Check sheet for the modelled part. Datum: model origin and axes. Units: mm. Round coordinates to 2 decimals unless told otherwise and drop trailing zeros. Write each loop counter-clockwise with the first axis right and the second up, starting at its lowest first coordinate (ties: lowest second). Pieces come first, ordered by that corner, then holes. Notation, with made-up numbers: (-21.5, 75.5) -> (7.5, 75.5) arc R18 ccw to (7.5, 81.5) -> close; hole circle Ø5 at (19, 6). An arc over 180 degrees is marked (long way). One line per item, written item: value.
from build123d import *

# Parameters (mm, degrees)
SALIENTE_EXTRUIR1_DEPTH = 10
SALIENTE_EXTRUIR2_DEPTH = 10
CROQUIS3_R              = 25
CORTAR_EXTRUIR1_DEPTH   = 10


with BuildPart() as part:
    # Croquis1 → Saliente-Extruir1 (new body)
    with BuildSketch(Plane(origin=(0, 0, 0), x_dir=(1, 0, 0), z_dir=(0, 1, 0))):
        with BuildLine():
            Line((-70, -70), (-70, 70))
            ThreePointArc((-70, 70), (-52.983030462, 76.249658661), (-44.055908755, 92.027554074))
            ThreePointArc((-44.055908755, 92.027554074), (-36.156795126, 78.313355526), (-21.147629234, 83.333333333))
            ThreePointArc((-21.147629234, 83.333333333), (0, 95), (21.147629234, 83.333333333))
            ThreePointArc((21.147629234, 83.333333333), (36.156795126, 78.313355526), (44.055908755, 92.027554074))
            ThreePointArc((44.055908755, 92.027554074), (52.983030462, 76.249658661), (70, 70))
            Line((70, 70), (70, -70))
            ThreePointArc((70, -70), (52.983030462, -76.249658661), (44.055908755, -92.027554074))
            ThreePointArc((44.055908755, -92.027554074), (36.156795126, -78.313355526), (21.147629234, -83.333333333))
            ThreePointArc((21.147629234, -83.333333333), (0, -95), (-21.147629234, -83.333333333))
            ThreePointArc((-21.147629234, -83.333333333), (-36.156795126, -78.313355526), (-44.055908755, -92.027554074))
            ThreePointArc((-44.055908755, -92.027554074), (-52.983030462, -76.249658661), (-70, -70))
        make_face()
    extrude(amount=SALIENTE_EXTRUIR1_DEPTH)

    # Croquis2 → Saliente-Extruir2 (add)
    with BuildSketch(Plane(origin=(0, 10, 0), x_dir=(1, 0, 0), z_dir=(0, 1, 0))):
        with BuildLine():
            Line((-70, 25.98076189), (-70, 70))
            ThreePointArc((-70, 70), (-85.909969357, 57.627811916), (-77.837993487, 39.160506523))
            ThreePointArc((-77.837993487, 39.160506523), (-72.107558403, 33.647896498), (-70, 25.98076189))
        make_face()
        with BuildLine():
            ThreePointArc((77.837993487, 39.160506523), (85.909969357, 57.627811916), (70, 70))
            Line((70, 70), (70, 25.98076213))
            ThreePointArc((70, 25.98076213), (72.107558465, 33.647896602), (77.837993487, 39.160506523))
        make_face()
        with BuildLine():
            ThreePointArc((77.5, 12.990381057), (72.009618939, 18.480762121), (70, 25.98076213))
            Line((70, 25.98076213), (70, -25.98076213))
            ThreePointArc((70, -25.98076213), (72.009618939, -18.480762121), (77.5, -12.990381057))
            ThreePointArc((77.5, -12.990381057), (85, 0), (77.5, 12.990381057))
        make_face()
        with BuildLine():
            Line((-70, -25.980762199), (-70, 25.98076189))
            ThreePointArc((-70, 25.98076189), (-72.009618999, 18.480762017), (-77.5, 12.990381057))
            ThreePointArc((-77.5, 12.990381057), (-85, 0), (-77.5, -12.990381057))
            ThreePointArc((-77.5, -12.990381057), (-72.009618922, -18.480762151), (-70, -25.980762199))
        make_face()
        with BuildLine():
            Line((-70, -70), (-70, -25.980762199))
            ThreePointArc((-70, -25.980762199), (-72.107558482, -33.647896631), (-77.837993487, -39.160506523))
            ThreePointArc((-77.837993487, -39.160506523), (-85.909969357, -57.627811916), (-70, -70))
        make_face()
        with BuildLine():
            ThreePointArc((77.837993487, -39.160506523), (72.107558465, -33.647896602), (70, -25.98076213))
            Line((70, -25.98076213), (70, -70))
            ThreePointArc((70, -70), (85.909969357, -57.627811916), (77.837993487, -39.160506523))
        make_face()
    extrude(amount=-SALIENTE_EXTRUIR2_DEPTH)

    # Croquis3 → Cortar-Extruir1 (cut)
    with BuildSketch(Plane(origin=(0, 10, 0), x_dir=(1, 0, 0), z_dir=(0, 1, 0))):
        with Locations(Location((0, 0, 0), (0, 0, 270))):
            Circle(CROQUIS3_R)
    extrude(amount=-CORTAR_EXTRUIR1_DEPTH, mode=Mode.SUBTRACT)


solid = part.part
Item 1: Sectioned sample at D-D (z = 43.5). Enter the section's corners in (x, y), then the cut area to 3 significant figures.
Result set:
outline: (-82.95, 0) -> (82.95, 0) -> (82.95, 10) -> (-82.95, 10) -> close
area: 1,660 mm^2
Item 2: Release check for a two-part mould opening along X. For faces 1 (the cylindrical face through (-52.786, 4.93, 76.418)), 2 (the cylindrical face through (36.38, 4.93, 78.4)), 3 (the cylindrical face through (53.181, 4.93, 76.083)) record: pulls with the +X half, pulls with the -X half, needs draft (parallel to the pull), parting line crosses it, or undercut.
Result set:
face 1: pulls with the -X half
face 2: undercut
face 3: pulls with the +X half
Item 3: Material ranges on line 1 along X through (y, z) = (9, -78.5); line 2 along Z through (x, y) = (-13, 2.5); line 3 along Z through (x, y) = (79, 2.5), recorded low to high.
Result set:
line 1: -50.64 to -36.62, -26.82 to 26.82, 36.62 to 50.64
line 2: -91.35 to -21.35, 21.35 to 91.35
line 3: -67.31 to -39.86, -12 to 12, 39.86 to 67.31
Item 4: Depth check by flat-ended pin: pin 1 (1.5 mm diameter, centred on y = 2.5, z = -2, fed in from -X); pin 2 (1.5 mm diameter, centred on x = 32, y = 1.5, fed in from +Z); pin 3 (5 mm diameter, centred on y = 1.5, z = -36.5, fed in from -X). Enter the tip coordinate at first touch or a pass-through.
Result set:
pin 1: x = -84.95
pin 2: z = 77.54
pin 3: x = -77.55
Item 5: Sectioned sample at C-C (y = 5.75). Enter the section's corners in (x, z), then the cut area to 3 significant figures.
Result set:
outline: (-77.84, -39.16) arc R16.42 ccw to (-70, -70) arc R26.29 cw to (-44.06, -92.03) arc R12.5 cw to (-21.15, -83.33) arc R25 ccw to (21.15, -83.33) arc R12.5 cw to (44.06, -92.03) arc R26.29 cw to (70, -70) arc R16.42 ccw to (77.84, -39.16) arc R15 cw to (77.5, -12.99) arc R15 ccw to (77.5, 12.99) arc R15 cw to (77.84, 39.16) arc R16.42 ccw to (70, 70) arc R26.29 cw to (44.06, 92.03) arc R12.5 cw to (21.15, 83.33) arc R25 ccw to (-21.15, 83.33) arc R12.5 cw to (-44.06, 92.03) arc R26.29 cw to (-70, 70) arc R16.42 ccw to (-77.84, 39.16) arc R15 cw to (-77.5, 12.99) arc R15 ccw to (-77.5, -12.99) arc R15 cw to start; hole circle Ø50 at (0, 0)
area: 23,500 mm^2
Item 6: Sectioned sample at B-B (z = 0). Enter the section's corners in (x, y).
Result set:
outline: (-85, 0) -> (-25, 0) -> (-25, 10) -> (-85, 10) -> close; (25, 0) -> (85, 0) -> (85, 10) -> (25, 10) -> close
Item 7: Sectioned sample at A-A (x = 0). Enter the section's corners in (y, z).
Result set:
outline: (0, -95) -> (10, -95) -> (10, -25) -> (0, -25) -> close; (0, 25) -> (10, 25) -> (10, 95) -> (0, 95) -> close
